The figure shows three views and two pictorial views of one solid part (mm, origin at its lowest corner). Answer the questions. A direction names the side the tool comes from. Coordinates: 2 decimals unless noted, no trailing zeros. Order: outer loops, then holes, each group sorted by start corner. A loop starts at its lowest first (then second) coordinate and runs counter-clockwise, first axis right, second up. Notation, with made-up numbers: (18.25, -39.75) -> (54.25, -39.75) arc R14 cw to (54.25, -32.75) -> close; hole circle Ø7 at (60.25, 66.25). An arc over 180 degrees is marked (long way). Return JSON: item names as keys, results as strings.
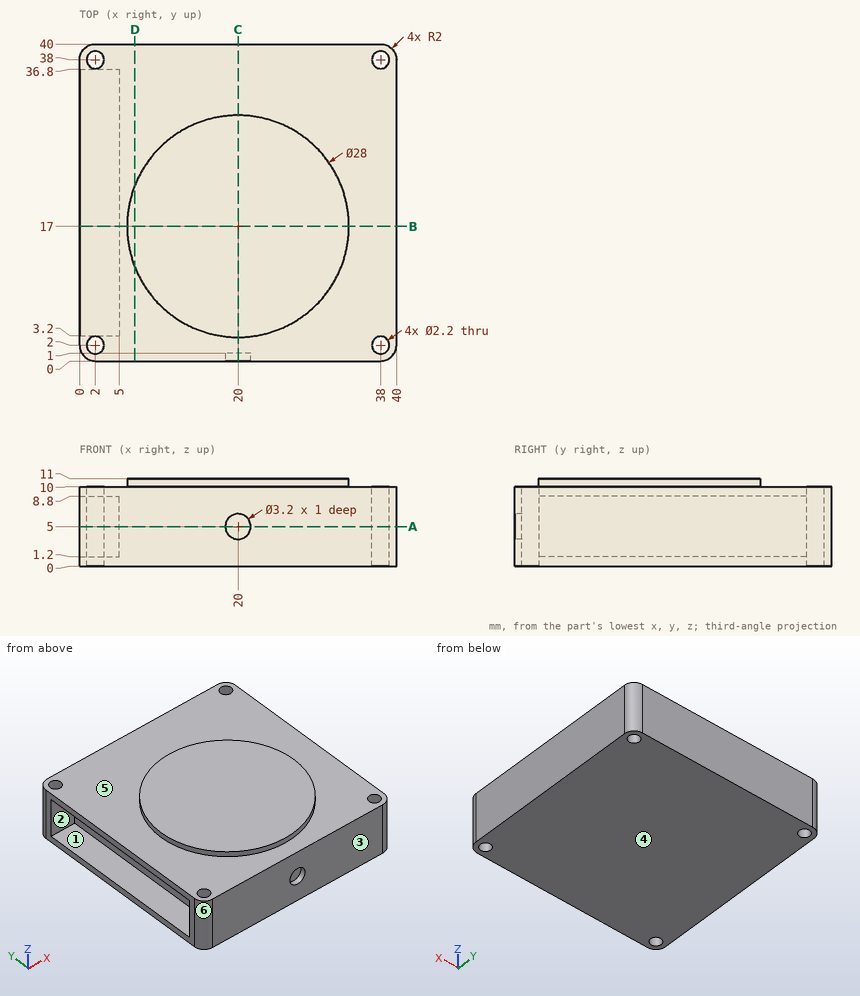
1. Each of these flat-tipped pins is pushed along its axis until it touches: pin 1 Ø2.5 at (y, z) = (24, 3) entering from -X; pin 2 Ø1.6 at (x, z) = (20.5, 4.5) entering from -Y; pin 3 Ø1.5 at (x, y) = (2, 27.5) entering from +Z. Where does it stop, or does it pass through?
Answer block:
{"pin 1": "stops at x = 5", "pin 2": "stops at y = 1", "pin 3": "stops at z = 10"}
2. Consider line 1 (X direction, y = 2, z = 3.75); line 2 (X direction, y = 3, z = 4.25). Determine where each line is inside the solid, lowest interval first. Write a range as from..to.
Answer block:
{"line 1": "x = 0..0.9, 3.1..36.9, 39.1..40", "line 2": "x = 0..1.54, 2.46..37.54, 38.46..40"}
3. The part is cut by section D-D on x = 7. Give the vertices of the cut face in (y, z).
Answer block:
{"outline": "(0, 0) -> (40, 0) -> (40, 10) -> (22.2, 10) -> (22.2, 11) -> (11.8, 11) -> (11.8, 10) -> (0, 10) -> close"}
4. The part is cut by section C-C on x = 20. Give the vertices of the cut face in (y, z), and give its area (3 significant figures).
Answer block:
{"outline": "(0, 0) -> (40, 0) -> (40, 10) -> (31, 10) -> (31, 11) -> (3, 11) -> (3, 10) -> (0, 10) -> (0, 6.6) -> (1, 6.6) -> (1, 3.4) -> (0, 3.4) -> close", "area": "425 mm2"}
5. For the marked faces 5 and 6, determine the directions among +Z, -Z, +X, -X, +Y, -Y from which every point of the face is accessible in a straight line to the end or side of a thin tool.
Answer block:
{"face 5": "+Z", "face 6": "+Z, -Z, -X, -Y"}
6. The part is cut by section B-B on y = 17. Give the vertices of the cut face in (x, z), and give its area (3 significant figures).
Answer block:
{"outline": "(0, 0) -> (40, 0) -> (40, 10) -> (34, 10) -> (34, 11) -> (6, 11) -> (6, 10) -> (0, 10) -> (0, 8.8) -> (5, 8.8) -> (5, 1.2) -> (0, 1.2) -> close", "area": "390 mm2"}
7. Determine the mould class of the marked faces 1, 2, 3 and 4 for opening direction Z: pulls with the +Z half, pulls with the -Z half, needs draft (parallel to the pull), parting line crosses it, or undercut.
Answer block:
{"face 1": "undercut", "face 2": "undercut", "face 3": "needs draft", "face 4": "pulls with the -Z half"}
8. The part is cut by section A-A on z = 5. Give the vertices of the cut face in (x, y).
Answer block:
{"outline": "(0, 2) arc R2 ccw to (2, 0) -> (18.4, 0) -> (18.4, 1) -> (21.6, 1) -> (21.6, 0) -> (38, 0) arc R2 ccw to (40, 2) -> (40, 38) arc R2 ccw to (38, 40) -> (2, 40) arc R2 ccw to (0, 38) -> (0, 36.8) -> (5, 36.8) -> (5, 3.2) -> (0, 3.2) -> close; hole circle Ø2.2 at (2, 2); hole circle Ø2.2 at (2, 38); hole circle Ø2.2 at (38, 2); hole circle Ø2.2 at (38, 38)"}
